from build123d import *

# Parameters (mm, degrees)
SKETCH1_W             = 32
SKETCH1_H             = 35
BRASS_BODY_DEPTH      = 30
COIL_START            = 30
SKETCH2_W             = 45
SKETCH2_H             = 40
COIL_DEPTH            = 30
INLET_STUB_START      = 17.5
SKETCH3_R             = 10.4775
INLET_STUB_DEPTH      = 20
OUTLET_STUB_START     = -37.5
SKETCH4_R             = 10.4775
OUTLET_STUB_DEPTH     = 20
INLET_BORE_START      = 37.5
SKETCH5_R             = 6
INLET_BORE_DEPTH      = 12
OUTLET_BORE_START     = -25.5
SKETCH6_R             = 6
OUTLET_BORE_DEPTH     = 12
SPADE_TERMINALS_START = 60
SKETCH7_W             = 0.8
SKETCH7_H             = 6.3
SPADE_TERMINALS_DEPTH = 8
FLOW_ARROW_START      = 16
FLOW_ARROW_DEPTH      = 0.6


with BuildPart() as part:
    # Sketch1 → Brass_Body (new body)
    with BuildSketch(Plane(origin=(0, 0, 0), x_dir=(1, 0, 0), z_dir=(0, 1, 0))):
        Rectangle(SKETCH1_W, SKETCH1_H)
    extrude(amount=BRASS_BODY_DEPTH)

    # Sketch2 → Coil (add)
    with BuildSketch(Plane(origin=(0, 0, 0), x_dir=(1, 0, 0), z_dir=(0, 1, 0)).offset(COIL_START)):
        Rectangle(SKETCH2_W, SKETCH2_H)
    extrude(amount=COIL_DEPTH)

    # Sketch3 → Inlet_Stub (add)
    with BuildSketch(Plane.XY.offset(INLET_STUB_START)):
        with Locations(Location((0, 15, 0), (0, 0, 180))):
            Circle(SKETCH3_R)
    extrude(amount=INLET_STUB_DEPTH)

    # Sketch4 → Outlet_Stub (add)
    with BuildSketch(Plane.XY.offset(OUTLET_STUB_START)):
        with Locations(Location((0, 15, 0), (0, 0, 180))):
            Circle(SKETCH4_R)
    extrude(amount=OUTLET_STUB_DEPTH)

    # Sketch5 → Inlet_Bore (cut)
    with BuildSketch(Plane.XY.offset(INLET_BORE_START)):
        with Locations((0, 15)):
            Circle(SKETCH5_R)
    extrude(amount=-INLET_BORE_DEPTH, mode=Mode.SUBTRACT)

    # Sketch6 → Outlet_Bore (cut)
    with BuildSketch(Plane.XY.offset(OUTLET_BORE_START)):
        with Locations((0, 15)):
            Circle(SKETCH6_R)
    extrude(amount=-OUTLET_BORE_DEPTH, mode=Mode.SUBTRACT)

    # Sketch7 → Spade_Terminals (add)
    with BuildSketch(Plane(origin=(0, 0, 0), x_dir=(1, 0, 0), z_dir=(0, 1, 0)).offset(SPADE_TERMINALS_START)):
        with Locations((-8, 0)):
            Rectangle(SKETCH7_W, SKETCH7_H)
        with Locations((8, 0)):
            Rectangle(SKETCH7_W, SKETCH7_H)
    extrude(amount=SPADE_TERMINALS_DEPTH)

    # Sketch8 → Flow_Arrow (add)
    with BuildSketch(Plane(origin=(0, 0, 0), x_dir=(0, 0, -1), z_dir=(1, 0, 0)).offset(FLOW_ARROW_START)):
        Polygon((-12, 9), (2, 9), (2, 6), (12, 12), (2, 18), (2, 15), (-12, 15), align=None)
    extrude(amount=FLOW_ARROW_DEPTH)


solid = part.part
Could you check a few things on this model? Use its own coordinates, in mm. A direction names the side the tool comes from. Give positions to 0.01 mm unless a question says otherwise; leave off trailing zeros. Loops run counter-clockwise (first coordinate to the right, second up) from the corner with the lowest first, then second, coordinate; pieces in that order, holes last. Notation, with made-up numbers: M -6,-20.75 L 36,-20.75 A17 ccw 36,-8.75 Z; hole C 87,20.5 d3. An arc over 180 degrees is marked long. Answer as a JSON object with one key per item and string values.
Q1. For faces 1 (the flat face through (7.6, 64, 0)), 2 (the cylindrical face through (2.27, 25.23, -27.64)), 3 (the flat face through (8.4, 64, 0)), which set-ups out of +Z, -Z, +X, -X, +Y, -Y let a thin tool reach every point of the face, with its end or its side?
Values found:
{"face 1": "+Z, -Z, +Y", "face 2": "-Z", "face 3": "+Z, -Z, +X, +Y"}
Q2. Suppose I cut it at D-D, the plane y = 17. List the corners of the cut face in (x, z) for me.
Values found:
{"outline": "M -16,-17.5 L -10.28,-17.5 L -10.28,-37.5 L -5.66,-37.5 L -5.66,-25.5 L 5.66,-25.5 L 5.66,-37.5 L 10.28,-37.5 L 10.28,-17.5 L 16,-17.5 L 16,-3.67 L 16.6,-3.67 L 16.6,-2 L 16,-2 L 16,17.5 L 10.28,17.5 L 10.28,37.5 L 5.66,37.5 L 5.66,25.5 L -5.66,25.5 L -5.66,37.5 L -10.28,37.5 L -10.28,17.5 L -16,17.5 Z"}
Q3. For P1, Ø12, axis at x = -17.5, y = 44.5, coming from the -Z side; P2, Ø6, axis at y = 25, z = 28, coming from the -X side; P3, Ø5, axis at y = 22.5, z = -10.5, coming from the +X side, each with a flat end and sliding along its axis, tell me the tip position at first contact or that it passes through.
Values found:
{"P1": "stops at z = -20", "P2": "stops at x = -7.8", "P3": "stops at x = 16"}
Q4. Suppose I cut it at B-B, the plane z = -11. List the corners of the cut face in (x, y) for me.
Values found:
{"outline": "M -22.5,30 L -16,30 L -16,0 L 16,0 L 16,11.4 L 16.6,11.4 L 16.6,12.6 L 16,12.6 L 16,30 L 22.5,30 L 22.5,60 L -22.5,60 Z"}
Q5. Suppose I cut it at A-A, the plane y = 63. List the corners of the cut face in (x, z) for me, plus the area to 3 significant figures.
Values found:
{"outline": "M -8.4,-3.15 L -7.6,-3.15 L -7.6,3.15 L -8.4,3.15 Z; M 7.6,-3.15 L 8.4,-3.15 L 8.4,3.15 L 7.6,3.15 Z", "area": "10.1 mm²"}
Q6. Suppose I cut it at C-C, the plane x = 0. List the corners of the cut face in (y, z) for me.
Values found:
{"outline": "M 0,-17.5 L 4.52,-17.5 L 4.52,-37.5 L 9,-37.5 L 9,-25.5 L 21,-25.5 L 21,-37.5 L 25.48,-37.5 L 25.48,-17.5 L 30,-17.5 L 30,-20 L 60,-20 L 60,20 L 30,20 L 30,17.5 L 25.48,17.5 L 25.48,37.5 L 21,37.5 L 21,25.5 L 9,25.5 L 9,37.5 L 4.52,37.5 L 4.52,17.5 L 0,17.5 Z"}
Q7. If we mould it in two halves opening along X, with no side actions, what happens to faces 4 (the cylindrical face through (2.27, 25.23, 27.36)), 5 (the flat face through (0, 15, -25.5)), 6 (the flat face through (0, 45, -20))? For each: pulls with the +X half, pulls with the -X half, needs draft (parallel to the pull), parting line crosses it, or undercut.
Values found:
{"face 4": "parting line crosses it", "face 5": "undercut", "face 6": "needs draft"}
Q8. If I drill on probe 1 along Y at (x, z) = (0, -33); probe 2 along Y at (x, z) = (19.5, 9.5); probe 3 along Z at (x, y) = (20.5, 42), over which ranges is the centre line in solid material (lowest first)? Write a range as [from, to].
Values found:
{"probe 1": "y = [4.52, 9], [21, 25.48]", "probe 2": "y = [30, 60]", "probe 3": "z = [-20, 20]"}
